Geometry: see drawing. Coordinates: mm, zero at the bounding-box minimum. Give positions to 0.01 mm unless a question says otherwise; leave off trailing zeros. Order: outer loops, then holes, each group sorted by start corner. A loop starts at its lowest first (then second) coordinate and runs counter-clockwise, first axis right, second up. Notation, with made-up numbers: (88, -28.5) - (134, -28.5) arc R14 cw to (134, -21.5) - close; hole circle Ø7 at (31.25, -35.75). An arc over 180 degrees is marked (long way). Put each result on its own line as item: value. Start each with the question number.
1. Section D-D on x = 0.95. Return the cut outline in (y, z), plus the area to 3 significant figures.
2. First-contact query: P1, Ø1, axis at x = 1, y = 2.5, coming from the +Z side. Flat tip, straight axial feed; report the tip coordinate or a pass-through.
3. Section B-B on y = 1.5. Return the cut outline in (x, z), plus the area to 3 significant figures.
4. Section A-A on x = 8.55. Return the cut outline in (y, z), plus the area to 3 significant figures.
5. Ray query, line 1 along Z through (x, y) = (3.5, 4.25); line 2 along Y through (x, z) = (4, 3.3); line 3 along X through (y, z) = (3, 2.3). Return the intervals inside material, ascending. Write a range as from..to.
6. Section C-C on z = 3.45. Return the cut outline in (x, y), plus the area to 3 significant figures.
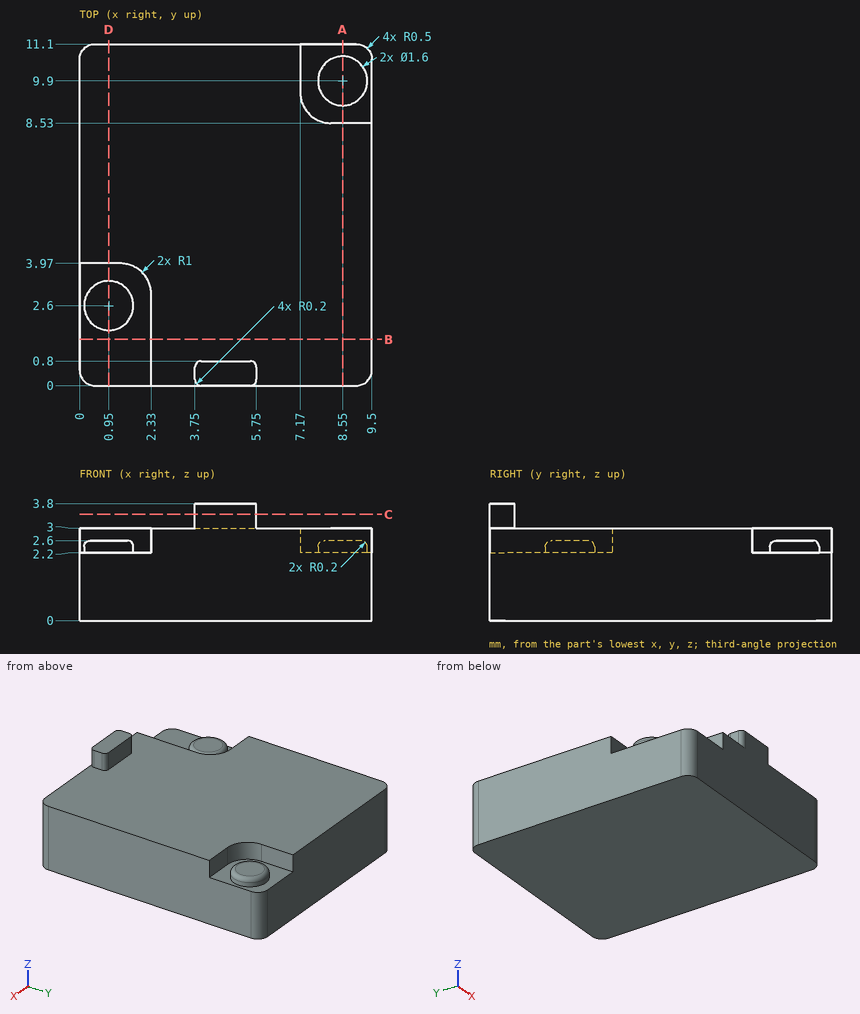
Resolved:
1. outline: (0, 0) - (11.1, 0) - (11.1, 3) - (3.97, 3) - (3.97, 2.2) - (3.4, 2.2) - (3.4, 2.4) arc R0.2 ccw to (3.2, 2.6) - (2, 2.6) arc R0.2 ccw to (1.8, 2.4) - (1.8, 2.2) - (0, 2.2) - close
1. area: 30.7 mm^2
2. P1: z = 2.6
3. outline: (0, 0) - (9.5, 0) - (9.5, 3) - (2.33, 3) - (2.33, 2.2) - (0, 2.2) - close
3. area: 26.6 mm^2
4. outline: (0, 0) - (11.1, 0) - (11.1, 2.2) - (10.7, 2.2) - (10.7, 2.4) arc R0.2 ccw to (10.5, 2.6) - (9.3, 2.6) arc R0.2 ccw to (9.1, 2.4) - (9.1, 2.2) - (8.53, 2.2) - (8.53, 3) - (0, 3) - close
4. area: 31.9 mm^2
5. line 1: 0..3
5. line 2: 0..0.8
5. line 3: 0.26..1.64, 2.33..9.5
6. outline: (3.75, 0.2) arc R0.2 ccw to (3.95, 0) - (5.55, 0) arc R0.2 ccw to (5.75, 0.2) - (5.75, 0.6) arc R0.2 ccw to (5.55, 0.8) - (3.95, 0.8) arc R0.2 ccw to (3.75, 0.6) - close
6. area: 1.57 mm^2
